Could you check a few things on this model? Use its own coordinates, in mm. Face numbers are marked on the shaded views. Give positions to 0.01 mm unless a question says otherwise; leave off trailing zeros. Loops run counter-clockwise (first coordinate to the right, second up) from the corner with the lowest first, then second, coordinate; pieces in that order, holes last. Notation, with made-up numbers: (62.25, 76.5) -> (91.25, 76.5) arc R19 ccw to (91.25, 85.5) -> close; hole circle Ø2 at (25.25, 13). An arc over 180 degrees is marked (long way). Write item = value, one per line. Start each with the question number.
1) I want a section at B-B (y = 7.5). List the corners of the cut face in (x, z) for me (3 decimals), and give its area (3 significant figures).
2) I want a section at A-A (z = 0). List the corners of the cut face in (x, y) for me (3 decimals).
3) If we mould it in two halves opening along X, with no side actions, what happens to the marked faces 1, 2 and 3? For each: +X half, -X half, draft (parallel to the pull), parting line (faces both ways), or undercut.
4) I want a section at C-C (x = 0). List the corners of the cut face in (y, z) for me (3 decimals), and give its area (3 significant figures).
5) I'm going to push a flat-ended pin straight in: pin 1 Ø3 at (x, z) = (5.5, 3) entering from -Y. Where does the tip first touch, or does it pass through?
6) I need wall thicknesses on probe 1 along Z at (x, y) = (0, 9.5) (3 decimals); probe 2 along Z at (x, y) = (-1.5, 14). Which ranges of each line are inside material? Lowest first, please. Write a range as from..to.
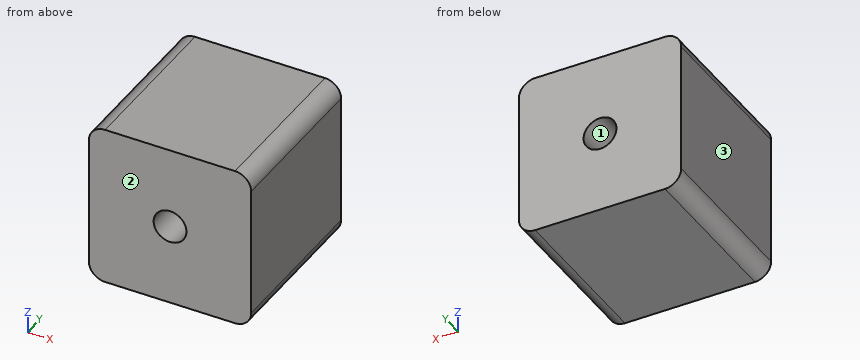
from build123d import *

# Parameters (mm, degrees)
SKETCH_1_W          = 20
SKETCH_1_H          = 20
EXTRUDE_1_DEPTH     = 20
SKETCH_2_R          = 2.025
CUT_EXTRUDE_1_DEPTH = 20
FILLET_1_R          = 2


with BuildPart() as part:
    # 草图1 → 凸台-拉伸1 (new body)
    with BuildSketch(Plane(origin=(0, 0, 0), x_dir=(1, 0, 0), z_dir=(0, 1, 0))):
        Rectangle(SKETCH_1_W, SKETCH_1_H)
    extrude(amount=EXTRUDE_1_DEPTH)

    # 草图2 → 切除-拉伸1 (cut)
    with BuildSketch(Plane(origin=(0, 20, 0), x_dir=(1, 0, 0), z_dir=(0, 1, 0))):
        Circle(SKETCH_2_R)
    extrude(amount=-CUT_EXTRUDE_1_DEPTH, mode=Mode.SUBTRACT)

    # 圆角1
    fillet_1_edges = [part.edges().sort_by_distance(p)[0] for p in [
        (10, 10, 10),
        (-10, 10, 10),
        (-10, 10, -10),
        (10, 10, -10),
    ]]
    fillet(fillet_1_edges, radius=FILLET_1_R)


solid = part.part
Answer list:
q1.outline = (-10, -8) arc R2 ccw to (-8, -10) -> (8, -10) arc R2 ccw to (10, -8) -> (10, 8) arc R2 ccw to (8, 10) -> (-8, 10) arc R2 ccw to (-10, 8) -> close; hole circle Ø4.05 at (0, 0)
q1.area = 384 mm^2
q2.outline = (-10, 0) -> (-2.025, 0) -> (-2.025, 20) -> (-10, 20) -> close; (2.025, 0) -> (10, 0) -> (10, 20) -> (2.025, 20) -> close
q3.face_1 = undercut
q3.face_2 = draft
q3.face_3 = -X half
q4.outline = (0, -10) -> (20, -10) -> (20, -2.025) -> (0, -2.025) -> close; (0, 2.025) -> (20, 2.025) -> (20, 10) -> (0, 10) -> close
q4.area = 319 mm^2
q5.pin_1 = 0
q6.probe_1 = -10..-2.025, 2.025..10
q6.probe_2 = -10..-1.36, 1.36..10
